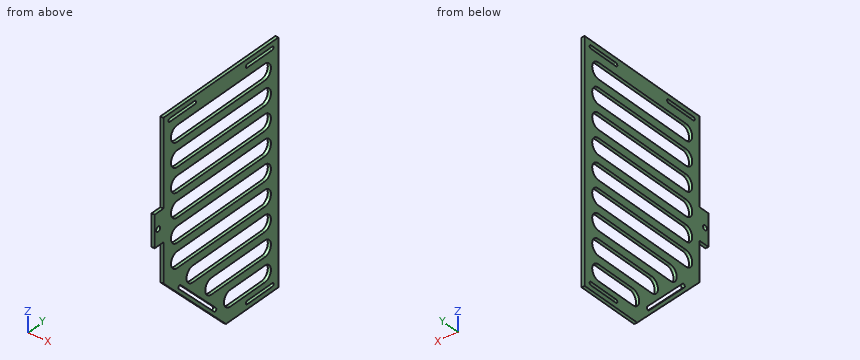
from build123d import *

# Parameters (mm, degrees)
SKETCH_2_W               = 148.55
SKETCH_2_H               = 92
EXTRUDE_1_DEPTH          = 2
CUT_EXTRUDE_1_DEPTH      = 88.388647003
CUT_EXTRUDE_1_DEPTH_BACK = 2
CUT_EXTRUDE_2_DEPTH      = 2
SKETCH_5_W               = 20
SKETCH_5_H               = 7
SKETCH_5_R               = 1.55
EXTRUDE_2_DEPTH          = 2
CUT_EXTRUDE_3_DEPTH      = 2
CUT_EXTRUDE_5_DEPTH      = 2


with BuildPart() as part:
    # 草图2 → 凸台-拉伸1 (new body)
    with BuildSketch(Plane(origin=(0, 0, 0), x_dir=(0, 0, -1), z_dir=(1, 0, 0))):
        Rectangle(SKETCH_2_W, SKETCH_2_H)
    extrude(amount=EXTRUDE_1_DEPTH)

    # 草图3 → 切除-拉伸1 (cut, two sides: drawn at the far end of the back side and taken through both)
    with BuildSketch(Plane(origin=(2, 0, 0), x_dir=(0, 0, -1), z_dir=(1, 0, 0)).offset(-CUT_EXTRUDE_1_DEPTH_BACK)):
        Polygon((-204.458434938, -274.733434938), (24.275, -46), (74.275, 4), (303.008434938, 232.733434938), (760.475304814, -224.733434938), (253.008434938, -732.200304814), align=None)
    extrude(amount=CUT_EXTRUDE_1_DEPTH + CUT_EXTRUDE_1_DEPTH_BACK, mode=Mode.SUBTRACT)

    # 草图4 → 切除-拉伸2 (cut)
    with BuildSketch(Plane(origin=(2, 0, 0), x_dir=(0, 0, -1), z_dir=(1, 0, 0))):
        with BuildLine():
            Line((-71.365, -41), (-71.365, -21))
            ThreePointArc((-71.365, -21), (-70.315, -19.95), (-69.265, -21))
            Line((-69.265, -21), (-69.265, -41))
            ThreePointArc((-69.265, -41), (-70.315, -42.05), (-71.365, -41))
        make_face()
        with BuildLine():
            Line((-71.365, 41), (-71.365, 21))
            ThreePointArc((-71.365, 21), (-70.315, 19.95), (-69.265, 21))
            Line((-69.265, 21), (-69.265, 41))
            ThreePointArc((-69.265, 41), (-70.315, 42.05), (-71.365, 41))
        make_face()
        with BuildLine():
            Line((71.365, 41), (71.365, 21))
            ThreePointArc((71.365, 21), (70.315, 19.95), (69.265, 21))
            Line((69.265, 21), (69.265, 41))
            ThreePointArc((69.265, 41), (70.315, 42.05), (71.365, 41))
        make_face()
    extrude(amount=-CUT_EXTRUDE_2_DEPTH, mode=Mode.SUBTRACT)

    # 草图5 → 凸台-拉伸2 (add)
    with BuildSketch(Plane(origin=(2, 0, 0), x_dir=(0, 0, -1), z_dir=(1, 0, 0))):
        with Locations((-10.315, -49.5)):
            Rectangle(SKETCH_5_W, SKETCH_5_H)
        with Locations((-10.315, -50.25)):
            Circle(SKETCH_5_R, mode=Mode.SUBTRACT)
    extrude(amount=-EXTRUDE_2_DEPTH)

    # 草图6 → 切除-拉伸3 (cut)
    with BuildSketch(Plane(origin=(2, 0, 0), x_dir=(0, 0, -1), z_dir=(1, 0, 0))):
        with BuildLine():
            Line((-64.275, -35), (-64.275, 35))
            ThreePointArc((-64.275, 35), (-59.275, 40), (-54.275, 35))
            Line((-54.275, 35), (-54.275, -35))
            ThreePointArc((-54.275, -35), (-59.275, -40), (-64.275, -35))
        make_face()
        with BuildLine():
            Line((-49.275, -35), (-49.275, 35))
            ThreePointArc((-49.275, 35), (-44.275, 40), (-39.275, 35))
            Line((-39.275, 35), (-39.275, -35))
            ThreePointArc((-39.275, -35), (-44.275, -40), (-49.275, -35))
        make_face()
        with BuildLine():
            Line((-34.275, -35), (-34.275, 35))
            ThreePointArc((-34.275, 35), (-29.275, 40), (-24.275, 35))
            Line((-24.275, 35), (-24.275, -35))
            ThreePointArc((-24.275, -35), (-29.275, -40), (-34.275, -35))
        make_face()
        with BuildLine():
            Line((-19.275, -35), (-19.275, 35))
            ThreePointArc((-19.275, 35), (-14.275, 40), (-9.275, 35))
            Line((-9.275, 35), (-9.275, -35))
            ThreePointArc((-9.275, -35), (-14.275, -40), (-19.275, -35))
        make_face()
        with BuildLine():
            Line((-4.275, -35), (-4.275, 35))
            ThreePointArc((-4.275, 35), (0.725, 40), (5.725, 35))
            Line((5.725, 35), (5.725, -35))
            ThreePointArc((5.725, -35), (0.725, -40), (-4.275, -35))
        make_face()
        with BuildLine():
            Line((10.725, -35), (10.725, 35))
            ThreePointArc((10.725, 35), (15.725, 40), (20.725, 35))
            Line((20.725, 35), (20.725, -35))
            ThreePointArc((20.725, -35), (15.725, -40), (10.725, -35))
        make_face()
        with BuildLine():
            Line((25.725, -22.579437252), (25.725, 35))
            ThreePointArc((25.725, 35), (30.725, 40), (35.725, 35))
            Line((35.725, 35), (35.725, -22.579437252))
            ThreePointArc((35.725, -22.579437252), (30.725, -27.579437252), (25.725, -22.579437252))
        make_face()
        with BuildLine():
            Line((40.725, -7.579437252), (40.725, 35))
            ThreePointArc((40.725, 35), (45.725, 40), (50.725, 35))
            Line((50.725, 35), (50.725, -7.579437252))
            ThreePointArc((50.725, -7.579437252), (45.725, -12.579437252), (40.725, -7.579437252))
        make_face()
        with BuildLine():
            Line((55.725, 7.420562748), (55.725, 35))
            ThreePointArc((55.725, 35), (60.725, 40), (65.725, 35))
            Line((65.725, 35), (65.725, 7.420562748))
            ThreePointArc((65.725, 7.420562748), (60.725, 2.420562748), (55.725, 7.420562748))
        make_face()
    extrude(amount=-CUT_EXTRUDE_3_DEPTH, mode=Mode.SUBTRACT)

    # 草图9 → 切除-拉伸5 (cut)
    with BuildSketch(Plane(origin=(2, 0, 0), x_dir=(0, 0, -1), z_dir=(1, 0, 0))):
        with BuildLine():
            Line((32.269081912, -32.27835316), (60.55335316, -3.994081912))
            ThreePointArc((60.55335316, -3.994081912), (62.0382774, -3.994081912), (62.0382774, -5.479006153))
            Line((62.0382774, -5.479006153), (33.754006153, -33.7632774))
            ThreePointArc((33.754006153, -33.7632774), (32.269081912, -33.7632774), (32.269081912, -32.27835316))
        make_face()
    extrude(amount=-CUT_EXTRUDE_5_DEPTH, mode=Mode.SUBTRACT)


solid = part.part
For this review, take the finished solid that the model builds, in its own axes (mm). Round coordinates to 2 decimals unless told otherwise and drop trailing zeros. Write each loop counter-clockwise with the first axis right and the second up, starting at its lowest first coordinate (ties: lowest second). Pieces come first, ordered by that corner, then holes. Notation, with made-up numbers: (15.25, 16.25) -> (32.25, 16.25) arc R23 cw to (32.25, 49.25) -> close; hole circle Ø10 at (52.5, 76.25). An arc over 180 degrees is marked (long way). Put each result on its own line as item: value.
Q1. Consider section C-C on z = -48.5. State the section outline as (x, y) points (3 decimals), and give its area (3 significant figures).
Determined:
outline: (0, -21.775) -> (2, -21.775) -> (2, -19.017) -> (0, -19.017) -> close; (0, -16.047) -> (2, -16.047) -> (2, -11.739) -> (0, -11.739) -> close; (0, 39.159) -> (2, 39.159) -> (2, 46) -> (0, 46) -> close
area: 27.8 mm^2
Q2. Clearance check with a flat-ended pin moving along its axis: pin 1 Ø1 at (x, y) = (1, -49.5) entering from +Z (3 decimals). State where the tip first meets the part, or that it passes through.
Determined:
pin 1: stops at z = 20.315
Q3. Consider section A-A on z = 17. State the section outline as (x, y) points.
Determined:
outline: (0, -53) -> (2, -53) -> (2, -39.19) -> (0, -39.19) -> close; (0, 39.19) -> (2, 39.19) -> (2, 46) -> (0, 46) -> close
Q4. To check wall thickness, follow L1, parallel to Y at x = 0.75, z = -23; L2, parallel to Y at x = 1.25, z = 2.5; L3, parallel to Y at x = 1.1, z = 60. State the ranges of each line that lie inside material, in increasing order. Write a range as [from, to].
Determined:
L1: y = [-46, 46]
L2: y = [-53, -38.82], [38.82, 46]
L3: y = [-46, -39.95], [39.95, 46]
Q5. Consider section B-B on y = 23.5. Give the number of separate pieces and of enclosed holes in the cut face, and give its area (3 significant figures).
Determined:
separate pieces: 12
enclosed holes: 0
area: 109 mm^2
